Geometry: final body of the model. Coordinates: model frame, mm. Give positions to 0.01 mm unless a question says otherwise; leave off trailing zeros. Write each loop counter-clockwise with the first axis right and the second up, starting at its lowest first coordinate (ties: lowest second). Pieces come first, ordered by that corner, then holes. Notation, with made-up numbers: (47.25, -7) -> (99.25, -7) arc R26 cw to (99.25, 10) -> close; hole circle Ø1 at (75.5, 61.25). An arc over 180 degrees is marked (long way). Answer as a JSON object with one key per item and string values. Group by question number.
(1) Draft query along X for faces 1 (the face through (362, 786, 0)), 2 (the face through (129.43, 1283.455, 5.07)). Return one class per face: +X half, -X half, draft (parallel to the pull), parting line (faces both ways), or undercut.
(2) Section query A-A on z = 5. Output: boundary loops of the cut face in (x, y), plus the area to 3 significant figures.
(3) Material intervals for probe 1 along Y at (x, z) = (6, 5); probe 2 along Y at (x, z) = (613, 7.25); probe 3 along Z at (x, y) = (6, 1755), sorted ascending.
(4) Section query C-C on y = 1556. Output: boundary loops of the cut face in (x, z), plus the area to 3 significant figures.
(5) Section query B-B on x = 367.5. Output: boundary loops of the cut face in (y, z).
(6) Contact query for a flat-ended pin moving along its axis: pin 1 Ø1.8 at (y, z) = (1754.5, 5) entering from -X. Output: stop coordinate, or through.
Autodesk Inventor part; units mm, degrees
ref_plane "Work Plane1" through (0, 992.5, 0) normal (0, 1, 0) x (-1, 0, 0)
ref_plane "YZ Plane" through (0, 0, 0) normal (1, 0, 0) x (0, 1, 0)
ref_plane "XY Plane" through (0, 0, 0) normal (0, 0, 1) x (1, 0, 0)
sketch "Sketch4" plane through (0, 0, 0) normal (0, 0, 1) x (1, 0, 0)
  line L0 (0, 0) -> (735, 0)
  line L1 (735, 0) -> (735, 1985)
  line L2 (735, 1985) -> (0, 1985)
  line L3 (0, 1985) -> (0, 0)
  dimension "d0" = 735
  dimension "d1" = 1985
extrude "Extrusion1" add sketch "Sketch4" along normal blind 10
sketch "Sketch5" plane through (0, 0, 10) normal (0, 0, 1) x (1, 0, 0)
  circle A0 centre (367.5, 1466) radius 300
  line L0 (735, 1985) -> (0, 1985)
  point P0 (0, 0)
  point P1 (367.5, 1985)
  dimension "d4" = 600
  dimension "d5" = 519
extrude "Extrusion2" cut sketch "Sketch5" against normal up to surface (10 mm away)
sketch "Sketch6" plane through (0, 0, 0) normal (0, 0, -1) x (-1, 0, 0)
  line L0 (-665, 720) -> (-665, 780) construction
  line L1 (-645, 720) -> (-645, 780)
  line L2 (-685, 780) -> (-685, 720)
  arc A0 (-685, 720) -> (-645, 720) centre (-665, 720) ccw
  arc A1 (-645, 780) -> (-685, 780) centre (-665, 780) ccw
  line L3 (0, 0) -> (-735, 0)
  line L4 (-735, 0) -> (-735, 1985)
  circle A2 centre (-665, 860) radius 3.5
  circle A3 centre (-665, 673) radius 3.5
  point P0 (-665, 750)
  point P1 (-665, 700)
  point P2 (-665, 800)
  dimension "d8" = 700
  dimension "d9" = 50
  dimension "d10" = 40
  dimension "d11" = 100
  dimension "d12" = 7
  dimension "d13" = 60
  dimension "d16" = 187
  dimension "d17" = 7
extrude "Extrusion3" cut sketch "Sketch6" against normal blind 10 contours A0 L2 A1 L1 | A2
extrude "Extrusion4" cut sketch "Sketch6" against normal up to surface (10 mm away) contours A3
sketch "Sketch7" plane through (0, 0, 0) normal (-1, 0, 0) x (0, 0, 1)
  circle A0 centre (5, 150) radius 3
  circle A1 centre (5, 230) radius 3
  line L0 (0, 0) -> (10, 0)
  point P0 (5, 0)
  dimension "d21" = 150
  dimension "d22" = 80
  dimension "d23" = 6
extrude "Extrusion5" cut sketch "Sketch7" against normal blind 15
thread "Thread1"
thread "Thread2"
ref_plane "Work Plane1" through (0, 992.5, 0) normal (0, 1, 0) x (-1, 0, 0)
mirror "Mirror1" about plane through (0, 992.5, 0) normal (0, 1, 0) of "Extrusion5"
equation "\"d0\" = RahmBrei"
equation "\"d1\" = RahmHoeh"
equation "\"d2\" = RahmDick"
equation "\"RahmBrei\" = 735"
equation "\"RahmHoeh\" = 1985"
equation "\"RahmDick\" = 10"
properties part number "Rahmen"
Answer list:
{
 "1": {"face 1": "draft", "face 2": "undercut"},
 "2": {"outline": "(0, 0) -> (735, 0) -> (735, 1985) -> (0, 1985) -> (0, 1838) -> (15, 1838) -> (15, 1832) -> (0, 1832) -> (0, 1758) -> (15, 1758) -> (15, 1752) -> (0, 1752) -> (0, 233) -> (15, 233) -> (15, 227) -> (0, 227) -> (0, 153) -> (15, 153) -> (15, 147) -> (0, 147) -> close; hole circle Ø600 at (367.5, 1466); hole (645, 720) arc R20 ccw to (685, 720) -> (685, 780) arc R20 ccw to (645, 780) -> close; hole circle Ø7 at (665, 673); hole circle Ø7 at (665, 860)", "area": "1,170,000 mm2"},
 "3": {"probe 1": "0 to 147, 153 to 227, 233 to 1752, 1758 to 1832, 1838 to 1985", "probe 2": "0 to 1293.58, 1638.42 to 1985", "probe 3": "0 to 2, 8 to 10"},
 "4": {"outline": "(0, 0) -> (81.32, 0) -> (81.32, 10) -> (0, 10) -> close; (653.68, 0) -> (735, 0) -> (735, 10) -> (653.68, 10) -> close", "area": "1,630 mm2"},
 "5": {"outline": "(0, 0) -> (1166, 0) -> (1166, 10) -> (0, 10) -> close; (1766, 0) -> (1985, 0) -> (1985, 10) -> (1766, 10) -> close"},
 "6": {"pin 1": "x = 15"}
}
